Can you work these out from the drawing? Everything is in mm from the part's minimum corner. A direction names the side the tool comes from. Coordinates: 2 decimals unless noted, no trailing zeros. Write each loop counter-clockwise with the first axis right and the second up, starting at its lowest first coordinate (ties: lowest second). Pieces come first, ordered by that corner, then holes. Notation, with made-up numbers: M 32,6 L 56,6 A27 cw 56,34 Z; hole C 20.5,71 d9. An arc over 180 degrees is marked long. Use one line per item in the form item = value. Start each with the question number.
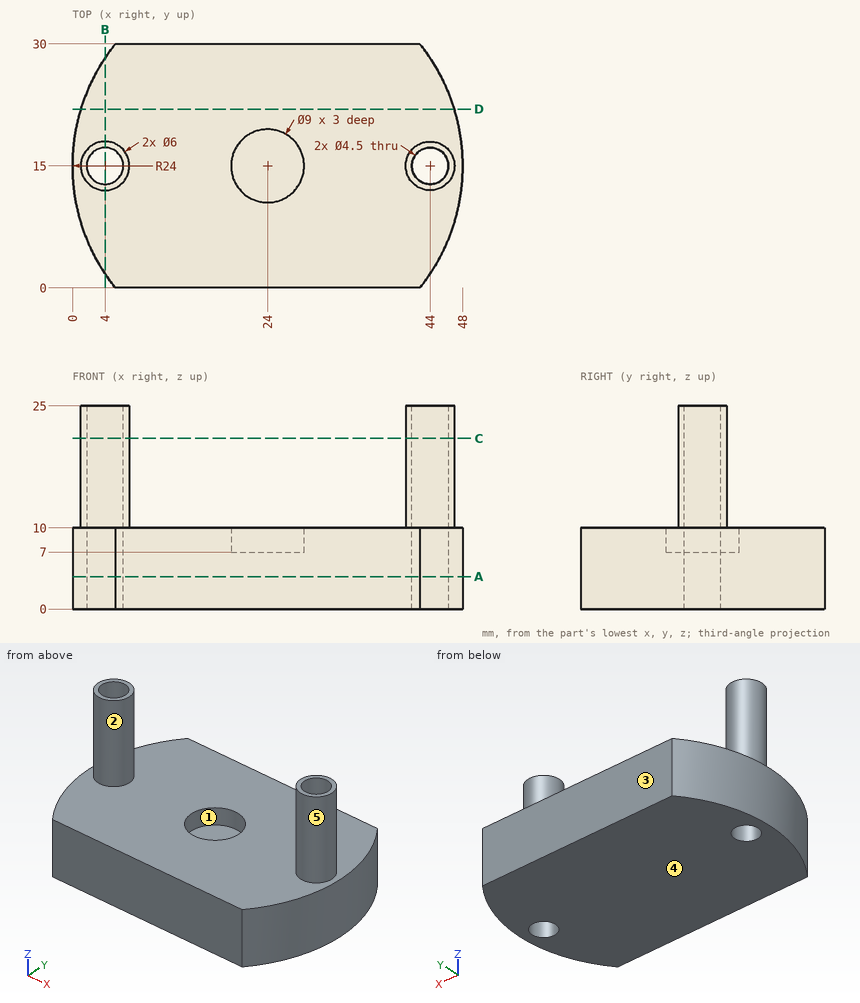
1) Suppose I cut it at C-C on z = 21. Please give me the cut outline in (x, y).
2) Suppose I cut it at A-A on z = 4. Please give me the cut outline in (x, y) (3 decimals).
3) Suppose I cut it at D-D on y = 22. Please give me the cut outline in (x, z).
4) Which directions (+Z, -Z, +X, -X, +Y, -Y) give clear straight access to the entire face, cutting with the end or side of a thin tool? Please do the marked faces 4 and 5.
5) Will these pins go through, and if not, where does the flat tip stop? pin 1 Ø8 at (x, z) = (33, 15) entering from -Y; pin 2 Ø6 at (x, y) = (4, 15) entering from +Z; pin 3 Ø1.5 at (y, z) = (7.5, 8.5) entering from -X; pin 4 Ø4.5 at (x, y) = (22.5, 13.5) entering from +Z.
6) Please list where these lines run through material, in increasing order: line 1 (X direction, y = 15, z = 20); line 2 (X direction, y = 15, z = 8.5); line 3 (X direction, y = 13, z = 2.25).
7) Suppose I cut it at B-B on x = 4. Please give me the cut outline in (y, z).
8) If we mould it in two halves opening along Y, with no side actions, what happens to the marked faces 1, 2 and 3? For each: +Y half, -Y half, draft (parallel to the pull), parting line (faces both ways), or undercut.
Computed values:
q1.outline = C 4,15 d6; C 44,15 d6; hole C 4,15 d4.5; hole C 44,15 d4.5
q2.outline = M 5.265,0 L 42.735,0 A24 ccw 42.735,30 L 5.265,30 A24 ccw Z; hole C 4,15 d4.5; hole C 44,15 d4.5
q3.outline = M 1.04,0 L 46.96,0 L 46.96,10 L 1.04,10 Z
q4.face_4 = -Z, +X, -X, +Y, -Y
q4.face_5 = +Z
q5.pin_1 = through
q5.pin_2 = 25
q5.pin_3 = 0.97
q5.pin_4 = 7
q6.line_1 = 1 to 1.75, 6.25 to 7, 41 to 41.75, 46.25 to 47
q6.line_2 = 0 to 1.75, 6.25 to 19.5, 28.5 to 41.75, 46.25 to 48
q6.line_3 = 0.08 to 2.97, 5.03 to 42.97, 45.03 to 47.92
q7.outline = M 1.73,0 L 12.75,0 L 12.75,25 L 12,25 L 12,10 L 1.73,10 Z; M 17.25,0 L 28.27,0 L 28.27,10 L 18,10 L 18,25 L 17.25,25 Z
q8.face_1 = undercut
q8.face_2 = parting line
q8.face_3 = +Y half
